```python
from build123d import *

# Parameters (mm, degrees)
SKETCH1_W           = 42.5
SKETCH1_H           = 42.5
SKETCH1_R           = 11.25
SKETCH1_R_2         = 1.65
BOSS_EXTRUDE1_DEPTH = 5
SKETCH3_W           = 10
SKETCH3_H           = 42.5
SKETCH3_W_2         = 5
SKETCH3_H_2         = 40
BOSS_EXTRUDE2_DEPTH = 25
CHAMFER1_SIZE       = 3
SKETCH5_W           = 40
SKETCH5_H           = 5
BOSS_EXTRUDE3_DEPTH = 15
CUT_EXTRUDE5_REACH  = 27
SKETCH9_R           = 2.25
CUT_EXTRUDE6_REACH  = 27
SKETCH10_R          = 2.25
SKETCH11_R          = 3.75
CUT_EXTRUDE7_DEPTH  = 1
SKETCH12_R          = 3.75
CUT_EXTRUDE8_DEPTH  = 1
CHAMFER2_SIZE       = 3


with BuildPart() as part:
    # Sketch1 → Boss-Extrude1 (new body)
    with BuildSketch(Plane(origin=(0, 0, 0), x_dir=(1, 0, 0), z_dir=(0, 1, 0))):
        Rectangle(SKETCH1_W, SKETCH1_H)
        Circle(SKETCH1_R, mode=Mode.SUBTRACT)
        with Locations((-15.5, 15.5)):
            Circle(SKETCH1_R_2, mode=Mode.SUBTRACT)
        with Locations((15.5, 15.5)):
            Circle(SKETCH1_R_2, mode=Mode.SUBTRACT)
        with Locations((15.5, -15.5)):
            Circle(SKETCH1_R_2, mode=Mode.SUBTRACT)
        with Locations((-15.5, -15.5)):
            Circle(SKETCH1_R_2, mode=Mode.SUBTRACT)
    extrude(amount=BOSS_EXTRUDE1_DEPTH)

    # Sketch3 → Boss-Extrude2 (add)
    with BuildSketch(Plane(origin=(0, 5, 0), x_dir=(1, 0, 0), z_dir=(0, 1, 0))):
        with Locations((26.25, 0)):
            Rectangle(SKETCH3_W, SKETCH3_H)
        with Locations((8.75, -41.25)):
            Rectangle(SKETCH3_W_2, SKETCH3_H_2)
    extrude(amount=-BOSS_EXTRUDE2_DEPTH)

    # Chamfer1
    chamfer1_edges = [part.edges().sort_by_distance(p)[0] for p in [
        (31.25, -7.5, -21.25),
        (31.25, -7.5, 21.25),
        (-21.25, 2.5, 21.25),
        (-21.25, 2.5, -21.25),
    ]]
    chamfer(chamfer1_edges, length=CHAMFER1_SIZE)

    # Sketch5 → Boss-Extrude3 (add)
    with BuildSketch(Plane.ZY.offset(-6.25)):
        with Locations((41.25, 2.5)):
            Rectangle(SKETCH5_W, SKETCH5_H)
    extrude(amount=BOSS_EXTRUDE3_DEPTH)

    # Sketch9 → Cut-Extrude5 (cut, up to next)
    with BuildSketch(Plane(origin=(0, 5, 0), x_dir=(1, 0, 0), z_dir=(0, 1, 0)), mode=Mode.PRIVATE) as cut_extrude5_sk1:
        with Locations((1.25, -51.25)):
            Circle(SKETCH9_R)
    cut_extrude5_tool1 = extrude(cut_extrude5_sk1.sketch, amount=-CUT_EXTRUDE5_REACH, mode=Mode.PRIVATE) & part.part
    add(cut_extrude5_tool1.solids().sort_by_distance((1.25, 5, 51.25))[0], mode=Mode.SUBTRACT)
    # Sketch9 → Cut-Extrude5 (cut, up to next)
    with BuildSketch(Plane(origin=(0, 5, 0), x_dir=(1, 0, 0), z_dir=(0, 1, 0)), mode=Mode.PRIVATE) as cut_extrude5_sk2:
        with Locations((1.25, -31.25)):
            Circle(SKETCH9_R)
    cut_extrude5_tool2 = extrude(cut_extrude5_sk2.sketch, amount=-CUT_EXTRUDE5_REACH, mode=Mode.PRIVATE) & part.part
    add(cut_extrude5_tool2.solids().sort_by_distance((1.25, 5, 31.25))[0], mode=Mode.SUBTRACT)

    # Sketch10 → Cut-Extrude6 (cut, up to next)
    with BuildSketch(Plane.ZY.offset(-6.25), mode=Mode.PRIVATE) as cut_extrude6_sk1:
        with Locations((51.25, -10)):
            Circle(SKETCH10_R)
    cut_extrude6_tool1 = extrude(cut_extrude6_sk1.sketch, amount=-CUT_EXTRUDE6_REACH, mode=Mode.PRIVATE) & part.part
    add(cut_extrude6_tool1.solids().sort_by_distance((6.25, -10, 51.25))[0], mode=Mode.SUBTRACT)
    # Sketch10 → Cut-Extrude6 (cut, up to next)
    with BuildSketch(Plane.ZY.offset(-6.25), mode=Mode.PRIVATE) as cut_extrude6_sk2:
        with Locations((31.25, -10)):
            Circle(SKETCH10_R)
    cut_extrude6_tool2 = extrude(cut_extrude6_sk2.sketch, amount=-CUT_EXTRUDE6_REACH, mode=Mode.PRIVATE) & part.part
    add(cut_extrude6_tool2.solids().sort_by_distance((6.25, -10, 31.25))[0], mode=Mode.SUBTRACT)

    # Sketch11 → Cut-Extrude7 (cut)
    with BuildSketch(Plane.XZ):
        with Locations((1.25, 51.25)):
            Circle(SKETCH11_R)
        with Locations((1.25, 31.25)):
            Circle(SKETCH11_R)
    extrude(amount=-CUT_EXTRUDE7_DEPTH, mode=Mode.SUBTRACT)

    # Sketch12 → Cut-Extrude8 (cut)
    with BuildSketch(Plane.ZY.offset(-6.25)):
        with Locations((31.25, -10)):
            Circle(SKETCH12_R)
        with Locations((51.25, -10)):
            Circle(SKETCH12_R)
    extrude(amount=-CUT_EXTRUDE8_DEPTH, mode=Mode.SUBTRACT)

    # Chamfer2
    chamfer2_edges = [part.edges().sort_by_distance(p)[0] for p in [
        (8.75, -20, 21.25),
        (8.75, -20, 61.25),
        (-8.75, 2.5, 61.25),
    ]]
    chamfer(chamfer2_edges, length=CHAMFER2_SIZE)


solid = part.part
```
Part model, mm, in its own coordinate system. A direction names the side the tool comes from. Give positions to 0.01 mm unless a question says otherwise; leave off trailing zeros. Write each loop counter-clockwise with the first axis right and the second up, starting at its lowest first coordinate (ties: lowest second). Pieces come first, ordered by that corner, then holes. Notation, with made-up numbers: M 46,79 L 73,79 A19 ccw 73,89 Z; hole C -8.5,34.5 d6. An arc over 180 degrees is marked long. Use CSV: the item, a comma, the result in double quotes.
Item 1: Slice it at B-B on x = -15.5. Write the cut outline in (y, z), plus the area to 4 significant figures.
Taken from the geometry:
outline,"M 0,-21.25 L 5,-21.25 L 5,-17.15 L 0,-17.15 Z; M 0,-13.85 L 5,-13.85 L 5,13.85 L 0,13.85 Z; M 0,17.15 L 5,17.15 L 5,21.25 L 0,21.25 Z"
area,"179.5 mm²"
Item 2: Slice it at A-A on y = -10. Write the cut outline in (x, z).
Taken from the geometry:
outline,"M 6.25,21.25 L 11.25,21.25 L 11.25,29 L 7.25,29 L 7.25,27.5 L 6.25,27.5 Z; M 6.25,35 L 7.25,35 L 7.25,33.5 L 11.25,33.5 L 11.25,49 L 7.25,49 L 7.25,47.5 L 6.25,47.5 Z; M 6.25,55 L 7.25,55 L 7.25,53.5 L 11.25,53.5 L 11.25,61.25 L 6.25,61.25 Z; M 21.25,-21.25 L 28.25,-21.25 L 31.25,-18.25 L 31.25,18.25 L 28.25,21.25 L 21.25,21.25 Z"
Item 3: Slice it at D-D on y = -2.25. Write the cut outline in (x, z), plus the area to 3 significant figures.
Taken from the geometry:
outline,"M 6.25,21.25 L 11.25,21.25 L 11.25,61.25 L 6.25,61.25 Z; M 21.25,-21.25 L 28.25,-21.25 L 31.25,-18.25 L 31.25,18.25 L 28.25,21.25 L 21.25,21.25 Z"
area,"616 mm²"
Item 4: Which spindle directions (+Z, -Z, +X, -X, +Y, -Y) get a long thin tool onto all of the face, cutting with end or side? Do faces 1 (the face through (9, -8, 21.25)), 2 (the face through (7.25, -12, 53)), 3 (the face through (11.25, -7, 42)), 4 (the face through (0.44, 0.49, 47.59)). Say none if no direction does.
Taken from the geometry:
face 1,"-Z, -X, -Y"
face 2,"-X"
face 3,"+Z, +X, +Y, -Y"
face 4,"-Y"
Item 5: Slice it at C-C on z = -15.5. Write the cut outline in (x, y), plus the area to 4 significant figures.
Taken from the geometry:
outline,"M -21.25,0 L -17.15,0 L -17.15,5 L -21.25,5 Z; M -13.85,0 L 13.85,0 L 13.85,5 L -13.85,5 Z; M 17.15,0 L 21.25,0 L 21.25,-20 L 31.25,-20 L 31.25,5 L 17.15,5 Z"
area,"429.5 mm²"
Item 6: Pull direction X, two halves, no side cores. Call faces 5 (the face through (12, 3, -21.25)), 6 (the face through (-21.25, 2, 0)), 7 (the face through (-13.926, 2.465, 15.004)): +X half, -X half, draft (parallel to the pull), parting line (faces both ways), or undercut.
Taken from the geometry:
face 5,"draft"
face 6,"-X half"
face 7,"undercut"
Item 7: Drill centre lines: probe 1 along X at (y, z) = (2.3, 15.5); probe 2 along Z at (x, y) = (15.5, 3.75); probe 3 along Z at (x, y) = (1.25, 0.4). Where is each one in solid material? Low to high.
Taken from the geometry:
probe 1,"x = -21.25 to -17.15, -13.85 to 13.85, 17.15 to 31.25"
probe 2,"z = -21.25 to -17.15, -13.85 to 13.85, 17.15 to 21.25"
probe 3,"z = -21.25 to -11.18, 11.18 to 27.5, 35 to 47.5, 55 to 61.25"
Item 8: Pin check, flat tips, straight feed: P1, Ø21, axis at x = -4.5, z = 39, coming from the -Y side; P2, Ø10, axis at y = -8.5, z = 10.5, coming from the -X side; P3, Ø2, axis at x = 2, z = 32.5, coming from the -Y side; P4, Ø20, axis at x = 0, z = 0, coming from the +Y side. Stop position of each tip, or through.
Taken from the geometry:
P1,"stops at y = 0"
P2,"stops at x = 21.25"
P3,"stops at y = 1"
P4,"passes through"
